Input: part model. Units: mm. Frame: model coordinates. A direction names the side the tool comes from. Give positions to 0.01 mm unless a question says otherwise; leave off trailing zeros. Loops run counter-clockwise (first coordinate to the right, second up) from the corner with the lowest first, then second, coordinate; pieces in that order, holes last. Notation, with made-up numbers: M 13,54 L 32,54 A21 ccw 32,61 Z; hole C 26.25,-9.5 d7. An arc over 180 degrees is marked long. Answer as a JSON object with one key per item and string values. Group by question number.
```python
from build123d import *

# Parameters (mm, degrees)
F5_DEPTH = 12.7


# Not quite as in the source:
# - a pattern or mirror of a feature is missing from the dataset's text; its kind, count and spacing are read off the source's solid


with BuildPart() as f1:
    # F0 (on Front) → F1 (revolve)
    with BuildSketch(Plane.XZ):
        with BuildLine():
            ThreePointArc((-23.0108623865, -28.5877), (-27.0923504321, -14.2949750325), (-23.01875, 0))
            Line((-23.01875, 0), (-30.2104195144, 0))
            ThreePointArc((-30.2104195144, 0), (-33.4185884522, -14.2945250314), (-30.20441, -28.5877))
            Line((-30.20441, -28.5877), (-23.0108623865, -28.5877))
        make_face()
    revolve(axis=Axis((0, 0, -13.0283376202), (0, 0, -1)))

    # F4 (on line) → F5 (cut)
    with BuildSketch(Plane(origin=(28.9413471977, 16.7092945953, 0), x_dir=(-0.5, 0.8660254038, 0), z_dir=(0.8660254038, 0.5, 0))):
        with BuildLine():
            Line((-6.6390036837, -22.225), (6.6390036837, -22.225))
            ThreePointArc((6.6390036837, -22.225), (10.34796, -14.2875), (6.6390036837, -6.35))
            Line((6.6390036837, -6.35), (-6.6390036837, -6.35))
            ThreePointArc((-6.6390036837, -6.35), (-10.34796, -14.2875), (-6.6390036837, -22.225))
        make_face()
    f5 = extrude(amount=-F5_DEPTH, mode=Mode.SUBTRACT)

    # F5_copies: F5 across plane
    add(f5.mirror(Plane(origin=(0, 0, 0), x_dir=(0.5, -0.8660254038, 0), z_dir=(-0.8660254038, -0.5, 0))), mode=Mode.SUBTRACT)


solid = f1.part
```
1. Section B-B (y = 13). Count the separate pieces of the cut face and the enclosed holes in it, then the cut area to 3 significant figures.
2. Section C-C (z = -10.25). Output: boundary loops of the cut face in (x, y), then the cut area to 3 significant figures.
3. Mould query, pull axis Z, two halves, no side actions, for faces 1 (the flat face through (-6.9, -22.2, 0)), 2 (the cylindrical face through (29.82, 5.27, -14.16)), 3 (the flat face through (6.9, -22.2, -28.588)). Classes: pulls with the +Z half, pulls with the -Z half, needs draft (parallel to the pull), parting line crosses it, or undercut.
4. Material intervals for L1, parallel to Z at x = -25, y = -13 (3 decimals); L2, parallel to Z at x = 17, y = 16.5; L3, parallel to Y at x = 14, z = -16, sorted ascending.
5. Section D-D (z = -24). Output: boundary loops of the cut face in (x, y).
6. Reachability of faces 4 (the cylindrical face through (-19.47, -23.19, -14.16)), 5 (the flat face through (25, 14, -22.225)), 6 (the cylindrical face through (19.47, 23.19, -14.41)), 7 (the cylindrical face through (-29.82, -5.27, -14.41)) from +Z, -Z, +X, -X, +Y, -Y: full face, straight path, thin tool, end or side. Return the list, or none.
7. Section A-A (x = -10). Output: boundary loops of the cut face in (y, z).
8. First-contact query: P1, Ø8, axis at x = -1, z = -9, coming from the -Y side; P2, Ø3, axis at y = -13.5, z = -3, coming from the -X side; P3, Ø8, axis at y = 21, z = -7, coming from the -X side. Flat tips, straight axial feed; report the tip coordinate or a pass-through.
Geometry results:
{
 "1": {"separate pieces": "3", "enclosed holes": "0", "area": "310 mm2"},
 "2": {"outline": "M -32.28,-7.64 L -26.45,-4.27 A26.79 cw 16.92,20.77 L 22.76,24.14 A33.17 ccw Z; M -22.76,-24.14 A33.17 ccw 32.28,7.64 L 26.45,4.27 A26.79 cw -16.92,-20.77 Z", "area": "955 mm2"},
 "3": {"face 1": "pulls with the +Z half", "face 2": "undercut", "face 3": "pulls with the -Z half"},
 "4": {"L1": "-28.588 to -22.225, -6.35 to 0", "L2": "-28.59 to -27.43, -1.14 to 0", "L3": "-30.3 to -23.13, 23.13 to 30.3"},
 "5": {"outline": "C 0,0 d63.95; hole C 0,0 d50.58"},
 "6": {"face 4": "-X", "face 5": "none", "face 6": "+X", "face 7": "-Y"},
 "7": {"outline": "M -28.51,0 A31.89 ccw -28.5,-28.59 L -20.72,-28.59 A25.18 cw -20.73,0 Z; M 20.72,-28.59 L 28.5,-28.59 A31.89 ccw 28.51,0 L 20.73,0 A25.18 cw Z"},
 "8": {"P1": "y = -33.39", "P2": "x = -29.29", "P3": "x = -28.01"}
}
